```python
from build123d import *

# Parameters (mm, degrees)
F1_R     = 12.5
F2_DEPTH = 25
F2_TAPER = -3
F3_R     = 1.7835138624
F4_DEPTH = 17
F7_DEPTH = 10


# Not quite as in the source:
# - a fillet or chamfer that OpenCascade refuses, or shapes differently, is made with other operations: its cross-section is extruded or revolved along the edge and cut away or added


with BuildPart() as f2:
    # F1 (on Top) → F2 (new body)
    with BuildSketch(Plane.XY):
        Circle(F1_R)
    extrude(amount=-F2_DEPTH, taper=F2_TAPER)

    # F3 (on offset) → F4 (cut)
    with BuildSketch(Plane.XY.offset(-3)):
        with Locations((0, -12.5270644203)):
            Circle(F3_R)
        with Locations((4.5252976236, -11.6811396879)):
            Circle(F3_R)
        with Locations((8.4394287276, -9.2576123132)):
            Circle(F3_R)
        with Locations((11.2137682175, -5.5837930974)):
            Circle(F3_R)
        with Locations((12.4736261719, -1.155851683)):
            Circle(F3_R)
        with Locations((12.0488517931, 3.4281939061)):
            Circle(F3_R)
        with Locations((9.9968132146, 7.5492429118)):
            Circle(F3_R)
        with Locations((6.5946496173, 10.6507248305)):
            Circle(F3_R)
        with Locations((2.3018420469, 12.3137673431)):
            Circle(F3_R)
        with Locations((-2.3018420469, 12.3137673431)):
            Circle(F3_R)
        with Locations((-6.5946496173, 10.6507248305)):
            Circle(F3_R)
        with Locations((-9.9968132146, 7.5492429118)):
            Circle(F3_R)
        with Locations((-12.0488517931, 3.4281939061)):
            Circle(F3_R)
        with Locations((-12.4736261719, -1.155851683)):
            Circle(F3_R)
        with Locations((-11.2137682175, -5.5837930974)):
            Circle(F3_R)
        with Locations((-8.4394287276, -9.2576123132)):
            Circle(F3_R)
        with Locations((-4.5252976236, -11.6811396879)):
            Circle(F3_R)
    extrude(amount=-F4_DEPTH, mode=Mode.SUBTRACT)

    # F5: fillet of radius 4 on 1 edges, made by hand

    # F5_s1 → F5_t2 (revolve, cut)
    with BuildSketch(Plane.XZ):
        with BuildLine():
            ThreePointArc((12.6986598722, -3.790656175), (11.4575600359, -1.098502516), (8.7041417331, 0))
            Line((8.7041417331, 0), (12.5, 0))
            Line((12.5, 0), (12.6986598722, -3.790656175))
        make_face()
    revolve(axis=Axis((0, 0, 0), (0, 0, -1)), mode=Mode.SUBTRACT)

    # F6 (on face) → F7 (cut)
    with BuildSketch(Plane(origin=(0, 0, -25), x_dir=(1, 0, 0), z_dir=(0, 0, -1))):
        with BuildLine():
            Line((-1.9557109083, -1.3185451265), (1.9557109083, -1.3185451265))
            ThreePointArc((1.9557109083, -1.3185451265), (0, 2.3586789539), (-1.9557109083, -1.3185451265))
        make_face()
    extrude(amount=-F7_DEPTH, mode=Mode.SUBTRACT)


solid = f2.part
```
Source: CAD feature listing. Evaluate the final solid. Frame: model axes, mm. A direction names the side the tool comes from. Round coordinates to 2 decimals unless told otherwise and drop trailing zeros. Loops run counter-clockwise (first coordinate to the right, second up) from the corner with the lowest first, then second, coordinate; pieces in that order, holes last.
1. Contact query for flat-ended pins moving along their axis: pin 1 (3 mm diameter, centred on y = -2, z = -20.5, fed in from -X); pin 2 (10 mm diameter, centred on y = -9, z = -13, fed in from -X); pin 3 (2.5 mm diameter, centred on x = -12, y = -0.5, fed in from +Z). Output: stop coordinate, or through.
2. Section query A-A on x = 0. Output: boundary loops of the cut face in (y, z).
3. Ray query, L1, parallel to X at y = 6.25, z = -11.5; L2, parallel to X at y = 10.5, z = -3.5; L3, parallel to X at y = 11.25, z = -10.25. Return the intervals inside material, ascending.
4. Mould query, pull axis Y, two halves, no side actions, for faces 4 (the cylindrical face through (0.053, -10.744, -11.381)), 5 (the flat face through (0, -3, -25)). Classes: released by +Y, released by -Y, zero draft, split by the parting line, or undercut.
5. Section query C-C on z = -22. Output: boundary loops of the cut face in (x, y).
6. Access query for faces 1 (the flat face through (-12, -1, -3)), 2 (the flat face through (-6, 10, -3)), 3 (the flat face through (0, -12, -3)). Directions: +Z, -Z, +X, -X, +Y, -Y. A direction counts if a zero-diameter tool reaches every point of the face in a straight line with its end or side. Return the directions, or none.
Answers below:
1. pin 1: stops at x = -13.6
1. pin 2: stops at x = -12.58
1. pin 3: stops at z = -0.57
2. outline: (-13.81, -25) - (-2.36, -25) - (-2.36, -15) - (1.32, -15) - (1.32, -25) - (13.81, -25) - (12.7, -3.79) arc R4 ccw to (8.7, 0) - (-8.7, 0) arc R4 ccw to (-12.58, -3) - (-10.74, -3) - (-10.74, -20) - (-13.55, -20) - close
3. L1: x = -11.52 to -11.22, -8.77 to 8.77, 11.22 to 11.52
3. L2: x = -4.82 to 4.82
3. L3: x = -4.91 to -3.73, -0.87 to 0.87, 3.73 to 4.91
4. face 4: undercut
4. face 5: zero draft
5. outline: circle Ø27.31 at (0, 0); hole (-1.96, 1.32) arc R2.36 ccw (long way) to (1.96, 1.32) - close
6. face 1: -X
6. face 2: none
6. face 3: -Y
